Model file for the job. Use its own axes, mm. A direction names the side the tool comes from. Coordinates: 2 decimals unless noted, no trailing zeros. Order: outer loops, then holes, each group sorted by start corner. A loop starts at its lowest first (then second) coordinate and runs counter-clockwise, first axis right, second up. Notation, with made-up numbers: (14, 28) -> (49, 28) arc R24 ccw to (49, 57) -> close; hole circle Ø8 at (58, 62.25). An arc over 180 degrees is marked (long way). Write item = value, one per line. Start each with the question number.
Q1. Wall check: line 1 (Y direction, x = 0, z = 1); line 2 (Z direction, x = 15.5, y = -8.5) (3 decimals); line 3 (X direction, y = -7.5, z = 23) (3 decimals). Give the ranges that are in metal, low to high. Write a range as from..to.
Q2. Cut at B-B, the plane y = -2.5. List the corners of the cut face in (x, z) (3 decimals).
Q3. 3-axis set-ups, long thin cutter, end or side, ignore diameter. For faces 4 (the face through (-30.495, -0.782, 1.191)), 5 (the face through (0, -4, 3.175)): which of +Z, -Z, +X, -X, +Y, -Y reach the whole face in a straight line?
Q4. Cut at C-C, the plane y = -8. List the corners of the cut face in (x, z) (3 decimals), plus the area to 3 significant figures.
Q5. Cut at D-D, the plane x = -22. List the corners of the cut face in (y, z) (1 decimal), plus the area to 3 significant figures.
Q6. Mould opens along X. For faces 1 (the face through (-10, -17.463, 3)), 2 (the face through (-3.233, -1.341, 1.565)), 3 (the face through (-31.75, -8, 16)) say: +X half, -X half, draft (parallel to the pull), parting line (faces both ways), or undercut.
Q7. Flat gauge pins, fed straight in: pin 1 (6 mm diameter, centred on x = -9.5, y = -12.5, fed in from -Z); pin 2 (4 mm diameter, centred on y = -6.5, z = 7.5, fed in from +X) (3 decimals); pin 3 (10 mm diameter, centred on x = 13, y = -1.5, fed in from +Z) (3 decimals). Where does each tip first touch, or does it go through?
Q8. Cut at A-A, the plane x = 0. List the corners of the cut face in (y, z) (1 decimal), plus the area to 3 significant figures.
from build123d import *

# Parameters (mm, degrees)
SKETCH2_W                    = 57.15
SKETCH2_H                    = 34.925
BASE_FLANGE1_DEPTH           = 3.175
SKETCH23_W                   = 57.15
SKETCH23_H                   = 2.02438
CUT_EXTRUDE3_DEPTH           = 34.638521909
M6_CLEARANCE_HOLE1_D         = 7
EDGE_FLANGE2_STRIP_W         = 14.7
EDGE_FLANGE2_STRIP_H         = 3.175
EDGE_FLANGE2_STRIP_CUT_DEPTH = 32.90062
EDGE_FLANGE2_DEPTH           = 32.90062
CUT_EXTRUDE2_DEPTH           = 79.817416579


# Sheet-metal steps are written as plain solids
with BuildPart() as part:
    # Sketch2 → Base-Flange1 (new body)
    with BuildSketch(Plane.XY):
        Rectangle(SKETCH2_W, SKETCH2_H)
    extrude(amount=BASE_FLANGE1_DEPTH)

    # Sketch23 → Cut-Extrude3 (cut, through all)
    with BuildSketch(Plane.XY.offset(3.175)):
        with Locations((0, 16.45031)):
            Rectangle(SKETCH23_W, SKETCH23_H)
    extrude(amount=-CUT_EXTRUDE3_DEPTH, mode=Mode.SUBTRACT)

    # M6 Clearance Hole1 (through all)
    with Locations(Plane.XY.offset(3.175)):
        with Locations((0, 0)):
            Hole(M6_CLEARANCE_HOLE1_D / 2)

    # Edge-Flange2 strip (across the edge) → Edge-Flange2 strip cut (cut)
    with BuildSketch(Plane(origin=(-28.575, 15.43812, 3.175), x_dir=(1, 0, 0), z_dir=(0, -1, 0))):
        with Locations((-6.35, -1.5875)):
            Rectangle(EDGE_FLANGE2_STRIP_W, EDGE_FLANGE2_STRIP_H)
    extrude(amount=EDGE_FLANGE2_STRIP_CUT_DEPTH, mode=Mode.SUBTRACT)

    # Edge-Flange2 section (across the edge) → Edge-Flange2 (add)
    with BuildSketch(Plane(origin=(-28.575, 15.43812, 3.175), x_dir=(1, 0, 0), z_dir=(0, -1, 0))):
        with BuildLine():
            Line((-3.175, 1), (-3.175, 44.45))
            Line((-3.175, 44.45), (0, 44.45))
            Line((0, 44.45), (0, 1))
            ThreePointArc((0, 1), (0.292893219, 0.292893219), (1, 0))
            Line((1, 0), (1, -3.175))
            ThreePointArc((1, -3.175), (-1.952170811, -1.952170811), (-3.175, 1))
        make_face()
    extrude(amount=EDGE_FLANGE2_DEPTH)

    # Sketch20 → Cut-Extrude2 (cut, through all)
    with BuildSketch(Plane.ZY.offset(31.75)):
        Polygon((4.175, 15.43812), (47.625, -17.4625), (47.625, 15.43812), align=None)
    extrude(amount=-CUT_EXTRUDE2_DEPTH, mode=Mode.SUBTRACT)


solid = part.part
Here are the results:
q1.line_1 = -17.46..-3.5, 3.5..15.44
q1.line_2 = 0..3.175
q1.line_3 = -31.75..-28.575
q2.outline = (-31.75, 4.175) arc R4.175 ccw to (-27.575, 0) -> (-2.449, 0) -> (-2.449, 3.175) -> (-27.575, 3.175) arc R1 cw to (-28.575, 4.175) -> (-28.575, 27.865) -> (-31.75, 27.865) -> close; (2.449, 0) -> (28.575, 0) -> (28.575, 3.175) -> (2.449, 3.175) -> close
q3.face_4 = -Z, -X, +Y, -Y
q3.face_5 = +Z, +X, +Y, -Y
q4.outline = (-31.75, 4.175) arc R4.175 ccw to (-27.575, 0) -> (28.575, 0) -> (28.575, 3.175) -> (-27.575, 3.175) arc R1 cw to (-28.575, 4.175) -> (-28.575, 35.128) -> (-31.75, 35.128) -> close
q4.area = 289 mm²
q5.outline = (-17.5, 0) -> (15.4, 0) -> (15.4, 3.2) -> (-17.5, 3.2) -> close
q5.area = 104 mm²
q6.face_1 = draft
q6.face_2 = undercut
q6.face_3 = -X half
q7.pin_1 = 0
q7.pin_2 = -28.575
q7.pin_3 = 3.175
q8.outline = (-17.5, 0) -> (-3.5, 0) -> (-3.5, 3.2) -> (-17.5, 3.2) -> close; (3.5, 0) -> (15.4, 0) -> (15.4, 3.2) -> (3.5, 3.2) -> close
q8.area = 82.2 mm²
